```python
from build123d import *

# Parameters (mm, degrees)
SKETCH_1_W          = 50
SKETCH_1_H          = 53
SKETCH_1_R          = 1.75
EXTRUDE_1_DEPTH     = 10
SKETCH_2_W          = 28
SKETCH_2_H          = 53
CUT_EXTRUDE_1_DEPTH = 3
CUT_EXTRUDE_2_DEPTH = 6
SKETCH_5_R          = 3
CUT_EXTRUDE_4_DEPTH = 3.2
SKETCH_6_W          = 10
SKETCH_6_H          = 26.5
EXTRUDE_2_DEPTH     = 30
SKETCH_7_W          = 5
SKETCH_7_H          = 26.5
CUT_EXTRUDE_5_DEPTH = 20
FILLET_2_R          = 10
FILLET_3_R          = 10
SKETCH_8_R          = 1.75
CUT_EXTRUDE_6_DEPTH = 20


with BuildPart() as part:
    # 草图1 → 凸台-拉伸1 (new body)
    with BuildSketch(Plane.XY):
        with Locations((25, -26.5)):
            Rectangle(SKETCH_1_W, SKETCH_1_H)
        with Locations((35, -22.5)):
            Circle(SKETCH_1_R, mode=Mode.SUBTRACT)
        with Locations((40.5, -15)):
            Circle(SKETCH_1_R, mode=Mode.SUBTRACT)
        with Locations((35, -37.5)):
            Circle(SKETCH_1_R, mode=Mode.SUBTRACT)
        with Locations(Location((15, -37.5, 0), (0, 0, 180))):
            Circle(SKETCH_1_R, mode=Mode.SUBTRACT)
        with Locations(Location((15, -22.5, 0), (0, 0, 180))):
            Circle(SKETCH_1_R, mode=Mode.SUBTRACT)
        with Locations(Location((9.5, -15, 0), (0, 0, 180))):
            Circle(SKETCH_1_R, mode=Mode.SUBTRACT)
    extrude(amount=EXTRUDE_1_DEPTH)

    # 草图2 → 切除-拉伸1 (cut)
    with BuildSketch(Plane.XY.offset(10)):
        with Locations((25, -26.5)):
            Rectangle(SKETCH_2_W, SKETCH_2_H)
    extrude(amount=-CUT_EXTRUDE_1_DEPTH, mode=Mode.SUBTRACT)

    # 草图3 → 切除-拉伸2 (cut)
    with BuildSketch(Plane.XY.offset(10)):
        Polygon((9.5, -18.464101615), (12.5, -16.732050808), (12.5, -13.267949192), (9.5, -11.535898385), (6.5, -13.267949192), (6.5, -16.732050808), align=None)
        Polygon((40.5, -18.464101615), (43.5, -16.732050808), (43.5, -13.267949192), (40.5, -11.535898385), (37.5, -13.267949192), (37.5, -16.732050808), align=None)
    extrude(amount=-CUT_EXTRUDE_2_DEPTH, mode=Mode.SUBTRACT)

    # 草图5 → 切除-拉伸4 (cut)
    with BuildSketch(Plane(origin=(0, 0, 0), x_dir=(-1, 0, 0), z_dir=(0, 0, -1))):
        with Locations((-35, -37.5)):
            Circle(SKETCH_5_R)
        with Locations((-35, -22.5)):
            Circle(SKETCH_5_R)
        with Locations((-15, -37.5)):
            Circle(SKETCH_5_R)
        with Locations((-15, -22.5)):
            Circle(SKETCH_5_R)
    extrude(amount=-CUT_EXTRUDE_4_DEPTH, mode=Mode.SUBTRACT)

    # 草图6 → 凸台-拉伸2 (add)
    with BuildSketch(Plane(origin=(0, 0, 0), x_dir=(-1, 0, 0), z_dir=(0, 0, -1))):
        with Locations((5, -13.25)):
            Rectangle(SKETCH_6_W, SKETCH_6_H)
    extrude(amount=-EXTRUDE_2_DEPTH)

    # 草图7 → 切除-拉伸5 (cut)
    with BuildSketch(Plane.XY.offset(30)):
        with Locations((-2.5, -13.25)):
            Rectangle(SKETCH_7_W, SKETCH_7_H)
    extrude(amount=-CUT_EXTRUDE_5_DEPTH, mode=Mode.SUBTRACT)

    # 圆角2
    fillet_2_edges = [part.edges().sort_by_distance(p)[0] for p in [
        (-7.5, 0, 30),
        (-7.5, -26.5, 30),
    ]]
    fillet(fillet_2_edges, radius=FILLET_2_R)

    # 圆角3
    # the kernel refuses this fillet: 10 mm, written as the material it adds along each edge
    with BuildSketch(Plane(origin=(0, -26.5, 0), x_dir=(-1, 0, 0), z_dir=(0, 0, 1))) as fillet_3_piece_1:
        with BuildLine():
            CenterArc((FILLET_3_R, FILLET_3_R), FILLET_3_R, 180, 90)
            Line((0, FILLET_3_R), (0, 0))
            Line((0, 0), (FILLET_3_R, 0))
        make_face()
    extrude(amount=10)

    # 草图8 → 切除-拉伸6 (cut)
    with BuildSketch(Plane(origin=(-5, 0, 0), x_dir=(0, 0, -1), z_dir=(1, 0, 0))):
        with Locations((-25, -13.25)):
            Circle(SKETCH_8_R)
    extrude(amount=-CUT_EXTRUDE_6_DEPTH, mode=Mode.SUBTRACT)


solid = part.part
```
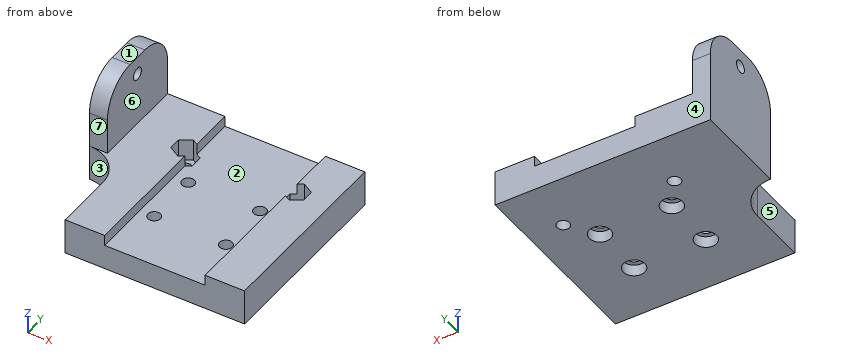
Can you work these out from the model? Positions are in its coordinate system, mm. Face numbers are marked on the shaded views. A direction names the side the tool comes from. Coordinates: 2 decimals unless noted, no trailing zeros. Loops run counter-clockwise (first coordinate to the right, second up) from the corner with the lowest first, then second, coordinate; pieces in that order, holes last. Notation, with made-up numbers: (65.5, 87.25) - (109.5, 87.25) arc R17 cw to (109.5, 93.25) - close; hole circle Ø7 at (0, 59). An arc over 180 degrees is marked (long way). Use a Markdown table: item, result.
Item 1: I want a section at C-C on z = 4.75. Please give me the cut outline in (x, y).
Numbers:
| item | result |
|---|---|
| outline | (-10, -26.5) arc R10 cw to (0, -36.5) - (0, -53) - (50, -53) - (50, 0) - (-10, 0) - close; hole (6.5, -16.73) - (9.5, -18.46) - (12.5, -16.73) - (12.5, -13.27) - (9.5, -11.54) - (6.5, -13.27) - close; hole circle Ø3.5 at (15, -37.5); hole circle Ø3.5 at (15, -22.5); hole circle Ø3.5 at (35, -37.5); hole circle Ø3.5 at (35, -22.5); hole (37.5, -16.73) - (40.5, -18.46) - (43.5, -16.73) - (43.5, -13.27) - (40.5, -11.54) - (37.5, -13.27) - close |
Item 2: For the marked faces 4, 5, 6 and 7, which set-ups out of +Z, -Z, +X, -X, +Y, -Y let a thin tool reach every point of the face, with its end or its side?
Numbers:
| item | result |
|---|---|
| face 4 | +Z, -Z, +X, -X, +Y |
| face 5 | +Z, -Z, -X, -Y |
| face 6 | +Z, +X, +Y, -Y |
| face 7 | +Z, +X, -X, -Y |
Item 3: If I drill on probe 1 along X at (y, z) = (-15, 2.8); probe 2 along X at (y, z) = (-47, 9.75); probe 3 along Y at (x, z) = (35, 6.1), over which ranges is the centre line in solid material (lowest first)? Write a range as from..to.
Numbers:
| item | result |
|---|---|
| probe 1 | x = -10..7.75, 11.25..38.75, 42.25..50 |
| probe 2 | x = 0..11, 39..50 |
| probe 3 | y = -53..-39.25, -35.75..-24.25, -20.75..0 |
Item 4: I want a section at D-D on z = 25. Please give me the cut outline in (x, y).
Numbers:
| item | result |
|---|---|
| outline | (-10, -25.16) - (-5, -25.16) - (-5, -15) - (-10, -15) - close; (-10, -11.5) - (-5, -11.5) - (-5, -1.34) - (-10, -1.34) - close |
Item 5: I want a section at B-B on x = 35. Please give me the cut outline in (y, z).
Numbers:
| item | result |
|---|---|
| outline | (-53, 0) - (-40.5, 0) - (-40.5, 3.2) - (-39.25, 3.2) - (-39.25, 7) - (-53, 7) - close; (-35.75, 3.2) - (-34.5, 3.2) - (-34.5, 0) - (-25.5, 0) - (-25.5, 3.2) - (-24.25, 3.2) - (-24.25, 7) - (-35.75, 7) - close; (-20.75, 3.2) - (-19.5, 3.2) - (-19.5, 0) - (0, 0) - (0, 7) - (-20.75, 7) - close |
Item 6: Will these pins go through, and if not, where does the flat tip stop? pin 1 (2 mm diameter, centred on x = 32.5, y = -11, fed in from +Z); pin 2 (6.5 mm diameter, centred on x = 9.5, y = -15, fed in from +Z).
Numbers:
| item | result |
|---|---|
| pin 1 | stops at z = 7 |
| pin 2 | stops at z = 10 |
Item 7: We'd pull the mould along X, two halves only. Please class the marked faces 1, 2 and 3: released by +X, released by -X, zero draft, split by the parting line, or undercut.
Numbers:
| item | result |
|---|---|
| face 1 | zero draft |
| face 2 | undercut |
| face 3 | released by -X |
Item 8: I want a section at A-A on y = -37.5. Please give me the cut outline in (x, z), and give its area (3 significant figures).
Numbers:
| item | result |
|---|---|
| outline | (0, 0) - (12, 0) - (12, 3.2) - (13.25, 3.2) - (13.25, 7) - (11, 7) - (11, 10) - (0, 10) - close; (16.75, 3.2) - (18, 3.2) - (18, 0) - (32, 0) - (32, 3.2) - (33.25, 3.2) - (33.25, 7) - (16.75, 7) - close; (36.75, 3.2) - (38, 3.2) - (38, 0) - (50, 0) - (50, 10) - (39, 10) - (39, 7) - (36.75, 7) - close |
| area | 351 mm2 |
